Check sheet for the drawn part. Datum: minimum x, y, z corner. Units: mm. Give positions to 0.01 mm unless a question says otherwise; leave off trailing zeros. Write each loop counter-clockwise with the first axis right and the second up, starting at its lowest first coordinate (ties: lowest second). Pieces come first, ordered by that corner, then holes. Notation, with made-up numbers: M 74.25,33.5 L 97.25,33.5 A29 ccw 97.25,70.5 Z; hole C 43.25,46.5 d7. An arc over 180 degrees is marked long. Write item = value, one per line. Start each with the question number.
1) Scan lines: L1, parallel to Y at x = 67, z = 0.75; L2, parallel to Y at x = 59.5, z = 1.4. Record each from-to range of solid material in increasing order.
2) Gauge pin test, flat end, axial feed: pin 1 (7 mm diameter, centred on x = 59.49, y = 59.49, fed in from +Z). Record the tip position at first contact, or that the pin passes through.
3) Sectioned sample at B-B, the plane z = 0.4. Count the separate pieces of the cut face and the enclosed holes in it, then the cut area to 3 significant figures.
4) Sectioned sample at A-A, the plane y = 67. Record the cut outline in (x, z).
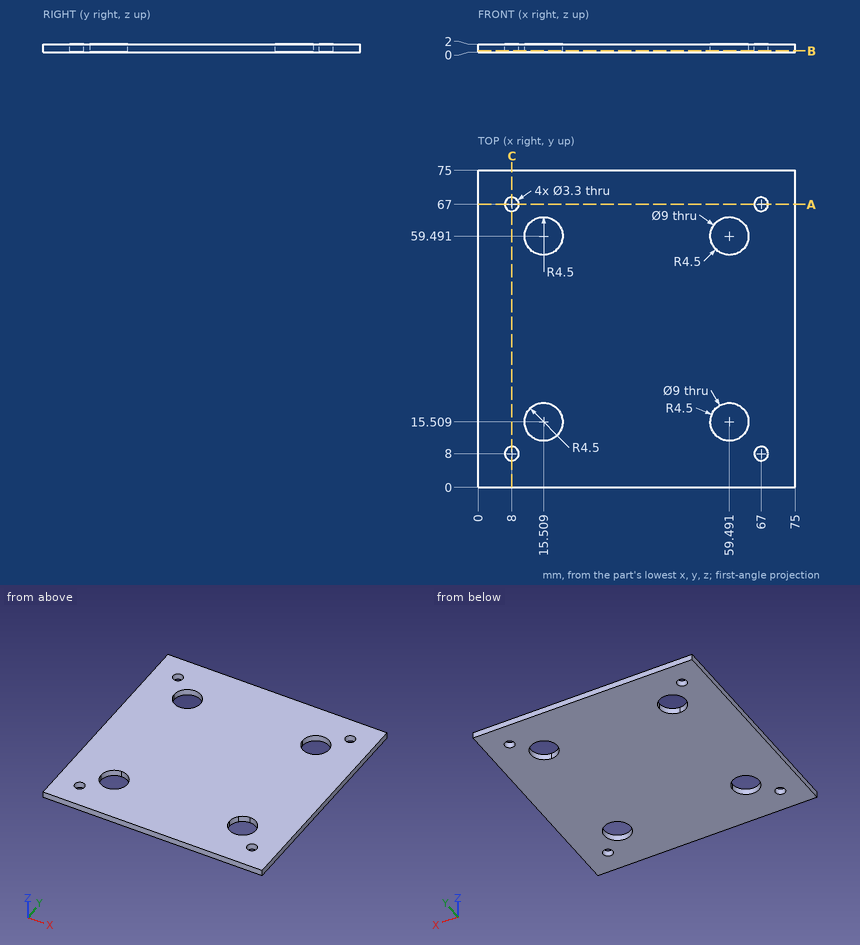
Data:
q1.L1 = 0 to 6.35, 9.65 to 65.35, 68.65 to 75
q1.L2 = 0 to 11.01, 20.01 to 54.99, 63.99 to 75
q2.pin_1 = through
q3.separate_pieces = 1
q3.enclosed_holes = 8
q3.area = 5,340 mm2
q4.outline = M 0,0 L 6.35,0 L 6.35,2 L 0,2 Z; M 9.65,0 L 65.35,0 L 65.35,2 L 9.65,2 Z; M 68.65,0 L 75,0 L 75,2 L 68.65,2 Z
